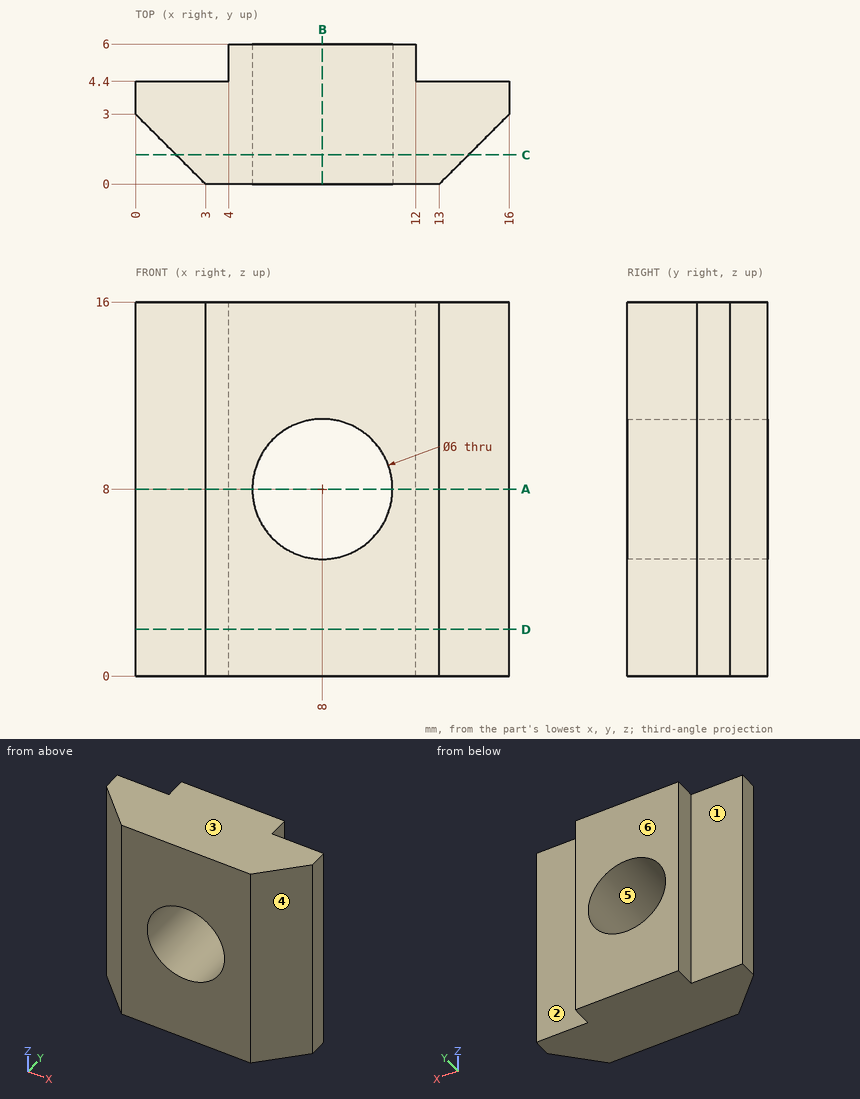
Study the drawing (mm; zero at the part's minimum x, y, z) and answer. A direction names the side the tool comes from. Round coordinates to 2 decimals unless told otherwise and drop trailing zeros. Loops run counter-clockwise (first coordinate to the right, second up) from the corner with the lowest first, then second, coordinate; pieces in that order, holes last. Notation, with made-up numbers: (-29.75, 73) -> (-5.75, 73) arc R13 ccw to (-5.75, 78) -> close; hole circle Ø8 at (51, 44.25). An arc over 180 degrees is marked (long way). Write each question's results on one line, items separated by ' | '. Start each with the question number.
1. Given pin 1 Ø4.5 at (x, z) = (1.5, 10) entering from +Y; pin 2 Ø4.5 at (x, z) = (14, 11.5) entering from +Y; pin 3 Ø1.8 at (y, z) = (5.5, 5) entering from +X, each flat-ended and moving along its own axis, determine where each tip first touches the part or whether it passes through.
2. A tool of negligible diameter and unlimited length cuts with its end or side. For the marked faces 1, 2 and 3, from which of +Z, -Z, +X, -X, +Y, -Y can it reach the whole face along a straight path? Write none if from no direction.
3. For a pull along X with two mould halves and no side action, classify the marked faces 4, 5 and 6 as +X half, -X half, draft (parallel to the pull), parting line (faces both ways), or undercut.
4. Section B-B (x = 8) is taken. Determine the outline of the cut face in (y, z), plus the area to 3 significant figures.
5. Section D-D (z = 2) is taken. Determine the outline of the cut face in (x, y).
6. Find the intervals of material crossed by probe 1 along X at (y, z) = (4.25, 8); probe 2 along X at (y, z) = (4.5, 4), in increasing order. Write a range as from..to.
7. Section C-C (y = 1.25) is taken. Determine the outline of the cut face in (x, z), plus the area to 3 significant figures.
8. Section A-A (z = 8) is taken. Determine the outline of the cut face in (x, y), plus the area to 3 significant figures.
Evaluation:
1) pin 1: stops at y = 4.4 | pin 2: stops at y = 6 | pin 3: stops at x = 12
2) face 1: +Z, -Z, -X, +Y | face 2: +Z, -Z, +X, +Y | face 3: +Z, +X, -X, +Y, -Y
3) face 4: +X half | face 5: undercut | face 6: draft
4) outline: (0, 0) -> (6, 0) -> (6, 5) -> (0, 5) -> close; (0, 11) -> (6, 11) -> (6, 16) -> (0, 16) -> close | area: 60.0 mm2
5) outline: (0, 3) -> (3, 0) -> (13, 0) -> (16, 3) -> (16, 4.4) -> (12, 4.4) -> (12, 6) -> (4, 6) -> (4, 4.4) -> (0, 4.4) -> close
6) probe 1: x = 0..5, 11..16 | probe 2: x = 4..12
7) outline: (1.75, 0) -> (14.25, 0) -> (14.25, 16) -> (1.75, 16) -> close; hole circle Ø6 at (8, 8) | area: 172 mm2
8) outline: (0, 3) -> (3, 0) -> (5, 0) -> (5, 6) -> (4, 6) -> (4, 4.4) -> (0, 4.4) -> close; (11, 0) -> (13, 0) -> (16, 3) -> (16, 4.4) -> (12, 4.4) -> (12, 6) -> (11, 6) -> close | area: 38.2 mm2
